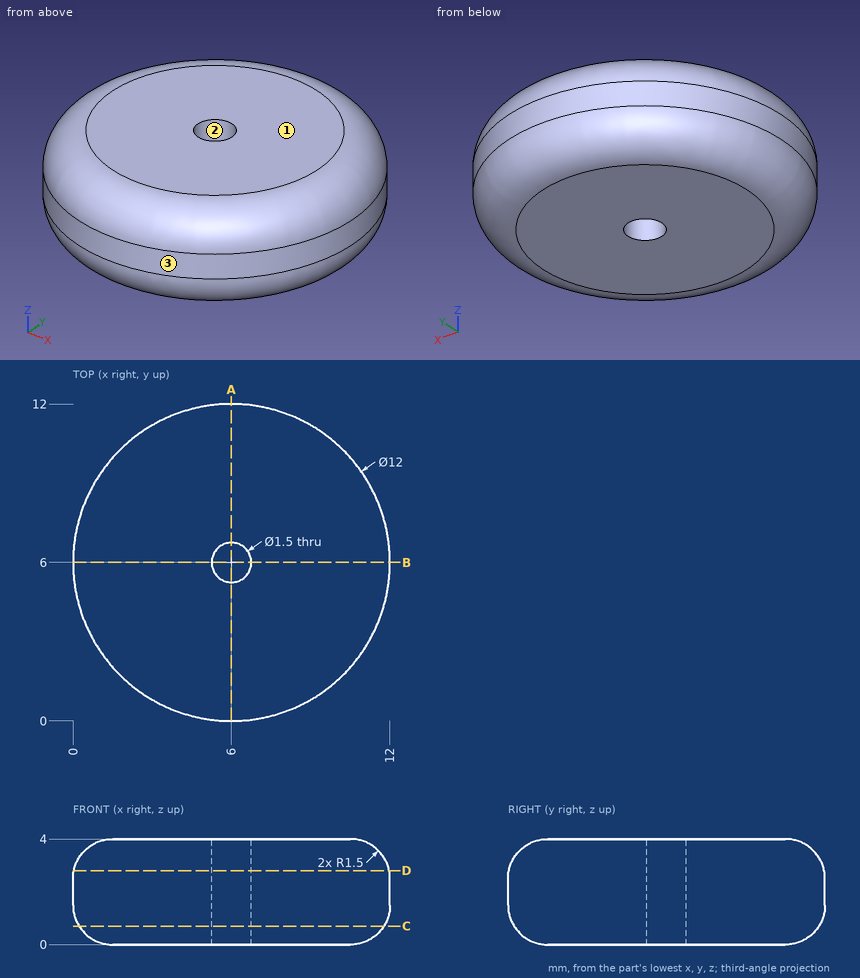
Part print with two shaded views. Sizes in mm from the minimum x, y, z corner. Round coordinates to 2 decimals unless told otherwise and drop trailing zeros. Loops run counter-clockwise (first coordinate to the right, second up) from the corner with the lowest first, then second, coordinate; pieces in that order, holes last.
1. Two-plate mould, pull along X, no slides. Class the marked faces 1, 2 and 3: pulls with the +X half, pulls with the -X half, needs draft (parallel to the pull), parting line crosses it, or undercut.
Solutions:
face 1: needs draft
face 2: undercut
face 3: parting line crosses it
2. Slice it at C-C (z = 0.7). Give the cut face in (x, y), and give its area (3 significant figures).
Solutions:
outline: circle Ø11.54 at (6, 6); hole circle Ø1.5 at (6, 6)
area: 103 mm2
3. Drill centre lines: line 1 along Y through (x, z) = (6, 1.7); line 2 along Y through (x, z) = (6, 3.15); line 3 along X through (y, z) = (5.75, 2.9). Where is each one in solid material? Low to high.
Solutions:
line 1: y = 0 to 5.25, 6.75 to 12
line 2: y = 0.15 to 5.25, 6.75 to 11.85
line 3: x = 0.06 to 5.29, 6.71 to 11.94
4. Slice it at D-D (z = 2.8). Give the cut face in (x, y).
Solutions:
outline: circle Ø11.94 at (6, 6); hole circle Ø1.5 at (6, 6)
5. Flat gauge pins, fed straight in: pin 1 (1.5 mm diameter, centred on y = 9, z = 3, fed in from +X); pin 2 (1 mm diameter, centred on x = 10.5, z = 3.5, fed in from +Y). Where does each tip first touch, or does it go through?
Solutions:
pin 1: stops at x = 11.52
pin 2: stops at y = 10.14
6. Slice it at A-A (x = 6). Give the cut face in (y, z).
Solutions:
outline: (0, 1.5) arc R1.5 ccw to (1.5, 0) - (5.25, 0) - (5.25, 4) - (1.5, 4) arc R1.5 ccw to (0, 2.5) - close; (6.75, 0) - (10.5, 0) arc R1.5 ccw to (12, 1.5) - (12, 2.5) arc R1.5 ccw to (10.5, 4) - (6.75, 4) - close
